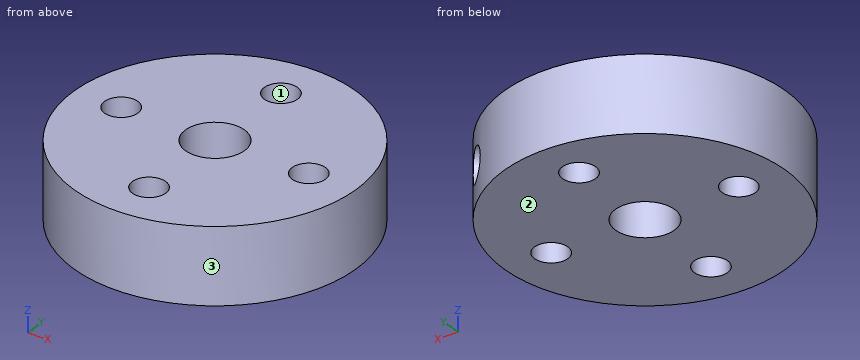
```python
from build123d import *

# Parameters (mm, degrees)
SKETCH1_R           = 9.525
SKETCH1_R_2         = 2
SKETCH1_R_3         = 1.1303
BOSS_EXTRUDE1_DEPTH = 5.08
SKETCH2_R           = 1.1303
CUT_EXTRUDE1_DEPTH  = 10.16


with BuildPart() as part:
    # Sketch1 → Boss-Extrude1 (new body)
    with BuildSketch(Plane.XY):
        Circle(SKETCH1_R)
        Circle(SKETCH1_R_2, mode=Mode.SUBTRACT)
        with Locations((-6.35, 0)):
            Circle(SKETCH1_R_3, mode=Mode.SUBTRACT)
        with Locations((0, 6.35)):
            Circle(SKETCH1_R_3, mode=Mode.SUBTRACT)
        with Locations((6.35, 0)):
            Circle(SKETCH1_R_3, mode=Mode.SUBTRACT)
        with Locations((0, -6.35)):
            Circle(SKETCH1_R_3, mode=Mode.SUBTRACT)
    extrude(amount=BOSS_EXTRUDE1_DEPTH)

    # Sketch2 → Cut-Extrude1 (cut)
    with BuildSketch(Plane(origin=(6.735192091, 6.735192091, 0), x_dir=(-0.707106781, 0.707106781, 0), z_dir=(0.707106781, 0.707106781, 0))):
        with Locations((0, 2.54)):
            Circle(SKETCH2_R)
    extrude(amount=-CUT_EXTRUDE1_DEPTH, mode=Mode.SUBTRACT)


solid = part.part
```
Geometry check sheet. Reference: the model listing, model coordinates, mm. Face numbers are marked on the shaded views. Give positions to 0.01 mm unless a question says otherwise; leave off trailing zeros. Loops run counter-clockwise (first coordinate to the right, second up) from the corner with the lowest first, then second, coordinate; pieces in that order, holes last. Notation, with made-up numbers: (3, 73) - (44, 73) arc R12 ccw to (44, 87) - close; hole circle Ø5 at (9.25, 6.25). An arc over 180 degrees is marked (long way). Use CSV: the item, a comma, the result in double quotes. Start each with the question number.
Q1. Scan lines: probe 1 along Y at (x, z) = (0, 3.15) (3 decimals); probe 2 along Y at (x, z) = (6.35, 1.8); probe 3 along Y at (x, z) = (6.35, 3.75). Record each from-to range of solid material in increasing order. Write a range as from..to.
Q2. Section check A-A, the plane x = -6.35. Record the cut outline in (y, z), and give its area (3 significant figures).
Q3. Release check for a two-part mould opening along Y. For the marked faces 1, 2 and 3 record: +Y half, -Y half, draft (parallel to the pull), parting line (faces both ways), or undercut.
Q4. Section check D-D, the plane y = 0.75. Count the separate pieces of the cut face and the enclosed holes in it, and give its area (3 significant figures).
Q5. Section check C-C, the plane z = 0.45. Record the cut outline in (x, y) (3 decimals), and give its area (3 significant figures).
Q6. Go/stop test with a flat-tipped pin: pin 1 Ø1 at (y, z) = (5, 2) entering from +X (3 decimals). Record where the tip stops, or that it passes through.
Findings below:
1,probe 1,"y = -9.525..-7.48, -5.22..-2, 2..5.22, 7.48..9.525"
1,probe 2,"y = -7.1..-1.13, 1.13..5.14"
1,probe 3,"y = -7.1..-1.13, 1.13..7.1"
2,outline,"(-7.1, 0) - (-1.13, 0) - (-1.13, 5.08) - (-7.1, 5.08) - close; (1.13, 0) - (7.1, 0) - (7.1, 5.08) - (1.13, 5.08) - close"
2,area,"60.6 mm^2"
3,face 1,"undercut"
3,face 2,"draft"
3,face 3,"parting line"
4,separate pieces,"4"
4,enclosed holes,"0"
4,area,"59.9 mm^2"
5,outline,"circle Ø19.05 at (0, 0); hole circle Ø2.261 at (-6.35, 0); hole circle Ø4 at (0, 0); hole circle Ø2.261 at (0, -6.35); hole circle Ø2.261 at (0, 6.35); hole circle Ø2.261 at (6.35, 0)"
5,area,"256 mm^2"
6,pin 1,"stops at x = 8.395"
